```python
from build123d import *

# Parameters (mm, degrees)
BOSS_EXTRUDE1_DEPTH = 6
SKETCH5_R           = 4
BOSS_EXTRUDE2_DEPTH = 1
BOSS_EXTRUDE3_DEPTH = 6
SKETCH6_R           = 2
CUT_EXTRUDE2_DEPTH  = 37.400549446
FILLET2_R           = 3
FILLET3_R           = 1.5
SKETCH3_R           = 1.75
CUT_EXTRUDE1_DEPTH  = 37.193922142
CUT_EXTRUDE3_REACH  = 38.401
SKETCH8_R           = 3
CHAMFER1_SIZE       = 1


with BuildPart() as part:
    # Sketch1 → Boss-Extrude1 (new, symmetric)
    with BuildSketch(Plane.XY):
        Polygon((-35, 0), (-35, 1), (-30, 2), (-25, 1), (0, 1), (0, 0), align=None)
    extrude(amount=BOSS_EXTRUDE1_DEPTH, both=True)

    # Sketch5 → Boss-Extrude2 (add)
    with BuildSketch(Plane.XZ):
        with Locations(Location((-20, 0, 0), (0, 0, 180))):
            Circle(SKETCH5_R)
    extrude(amount=BOSS_EXTRUDE2_DEPTH)

    # Sketch7 → Boss-Extrude3 (add, symmetric)
    with BuildSketch(Plane.XY):
        Polygon((0, 1), (0, 7), (-35, 7), (-35, 4), (-8, 4), (-8, 1), align=None)
    extrude(amount=BOSS_EXTRUDE3_DEPTH, both=True)

    # Sketch6 → Cut-Extrude2 (cut, through all)
    with BuildSketch(Plane.XZ.offset(1)):
        with Locations((-20, 0)):
            Circle(SKETCH6_R)
    extrude(amount=-CUT_EXTRUDE2_DEPTH, mode=Mode.SUBTRACT)

    # Fillet2
    fillet2_edges = [part.edges().sort_by_distance(p)[0] for p in [
        (-30, 2, 0),
    ]]
    fillet(fillet2_edges, radius=FILLET2_R)

    # Fillet3
    fillet3_edges = [part.edges().sort_by_distance(p)[0] for p in [
        (-8, 4, 0),
        (-8, 1, 0),
    ]]
    fillet(fillet3_edges, radius=FILLET3_R - 0.0001)  # a hair under: the kernel refuses the full size

    # Mirror1: part across plane


with BuildPart() as part_1:
    add(part.part)
    add(part.part.mirror(Plane(origin=(0, 0, 0), x_dir=(0, 0, 1), z_dir=(1, 0, 0))))

    # Sketch3 → Cut-Extrude1 (cut, through all)
    with BuildSketch(Plane(origin=(0, 0, 0), x_dir=(1, 0, 0), z_dir=(0, 1, 0))):
        with Locations(Location((0, 0, 0), (0, 0, 270))):
            Circle(SKETCH3_R)
    extrude(amount=CUT_EXTRUDE1_DEPTH, mode=Mode.SUBTRACT)

    # Sketch8 → Cut-Extrude3 (cut, up to next)
    with BuildSketch(Plane(origin=(0, 7, 0), x_dir=(1, 0, 0), z_dir=(0, 1, 0)), mode=Mode.PRIVATE) as cut_extrude3_sk1:
        with Locations(Location((20, 0, 0), (0, 0, 180))):
            Circle(SKETCH8_R)
    cut_extrude3_tool1 = extrude(cut_extrude3_sk1.sketch, amount=-CUT_EXTRUDE3_REACH, mode=Mode.PRIVATE) & part_1.part
    # Sketch8 → Cut-Extrude3 (cut, up to next)
    with BuildSketch(Plane(origin=(0, 7, 0), x_dir=(1, 0, 0), z_dir=(0, 1, 0)), mode=Mode.PRIVATE) as cut_extrude3_sk2:
        with Locations(Location((-20, 0, 0), (0, 0, 180))):
            Circle(SKETCH8_R)
    cut_extrude3_tool2 = extrude(cut_extrude3_sk2.sketch, amount=-CUT_EXTRUDE3_REACH, mode=Mode.PRIVATE) & part_1.part
    add(cut_extrude3_tool1.solids().sort_by_distance((20, 7, 0))[0], mode=Mode.SUBTRACT)
    add(cut_extrude3_tool2.solids().sort_by_distance((-20, 7, 0))[0], mode=Mode.SUBTRACT)

    # Chamfer1
    chamfer1_edges = [part_1.edges().sort_by_distance(p)[0] for p in [
        (-16, -1, 0),
        (16, -1, 0),
    ]]
    chamfer(chamfer1_edges, length=CHAMFER1_SIZE - 0.0001)  # a hair under: the kernel refuses the full size


solid = part_1.part
```
The model under review builds one solid part; all positions refer to its coordinate system, in mm. A direction names the side the tool comes from. Coordinates: 2 decimals unless noted, no trailing zeros. Write each loop counter-clockwise with the first axis right and the second up, starting at its lowest first coordinate (ties: lowest second). Pieces come first, ordered by that corner, then holes. Notation, with made-up numbers: (55, 68.25) - (80, 68.25) arc R37 cw to (80, 106.25) - close; hole circle Ø7 at (68.25, 38.25). An arc over 180 degrees is marked (long way). Answer in a Markdown table with one row per item. Add a question column.
Q1. Consider section A-A on x = -26. Give the boundary of the cut face in (y, z).
Q2. Consider section B-B on z = 0. Give the number of separate pieces and of enclosed holes in the cut face, then the cut area to 3 significant figures.
Q3. Clearance check with a flat-ended pin moving along its axis: pin 1 (6 mm diameter, centred on x = -7.5, z = 0, fed in from -Y). State where the tip first meets the part, or that it passes through.
Q4. For faces 1 (the face through (8.45, 1.43, -0.08)), 2 (the face through (-25, 4, 0)), 3 (the face through (32.825, 1.435, 0.084)), list the 3-axis set-ups (+Z, -Z, +X, -X, +Y, -Y) from which the entire face can be reached by the end or side of a thin tool; tool diameter is ignored.
Q5. Consider section C-C on x = 0. Give the boundary of the cut face in (y, z).
Q6. Draft analysis for pull direction X (two halves, no side actions). For faces 4 (the face through (0, 7, 3)), 5 (the face through (-8.43, 3.55, -0.08)), 6 (the face through (17, 1, 0)), state which applies: +X half, -X half, draft (parallel to the pull), parting line (faces both ways), or undercut.
Q7. To check wall thickness, follow line 1 along Y through (x, z) = (-16.5, -2.5); line 2 along X through (y, z) = (5.25, -1); line 3 along X through (y, z) = (5.5, 2.75). State the ranges of each line that lie inside material, in increasing order. Write a range as from..to.
Answers below:
| question | item | result |
|---|---|---|
| 1 | outline | (0, -6) - (1.2, -6) - (1.2, 6) - (0, 6) - close; (4, -6) - (7, -6) - (7, 6) - (4, 6) - close |
| 2 | separate pieces | 6 |
| 2 | enclosed holes | 0 |
| 2 | area | 277 mm² |
| 3 | pin 1 | y = 0 |
| 4 | face 1 | +Z, -Z |
| 4 | face 2 | +Z, -Z, -X |
| 4 | face 3 | +Z, -Z, +X |
| 5 | outline | (0, -6) - (7, -6) - (7, -1.75) - (0, -1.75) - close; (0, 1.75) - (7, 1.75) - (7, 6) - (0, 6) - close |
| 6 | face 4 | draft |
| 6 | face 5 | -X half |
| 6 | face 6 | undercut |
| 7 | line 1 | 0..1, 4..7 |
| 7 | line 2 | -35..-22.83, -17.17..-1.44, 1.44..17.17, 22.83..35 |
| 7 | line 3 | -35..-21.2, -18.8..18.8, 21.2..35 |
